CAD build for the part. Positions are in the model's coordinates, mm. Face numbers are marked on the shaded views. A direction names the side the tool comes from. Round coordinates to 2 decimals unless told otherwise and drop trailing zeros. Write each loop counter-clockwise with the first axis right and the second up, starting at its lowest first coordinate (ties: lowest second). Pieces come first, ordered by that corner, then holes. Notation, with made-up numbers: (17, -26) - (42, -26) arc R4 ccw to (42, -19) - close; hole circle Ø3 at (81, 47). An arc over 180 degrees is marked (long way). Answer in a Markdown table with one row per item.
```python
from build123d import *

# Parameters (mm, degrees)
F0_R     = 1.5875
F1_DEPTH = 38.1
F2_DEPTH = 40.64


with BuildPart() as f1:
    # F0 (on Front) → F1 (new body)
    with BuildSketch(Plane.XZ):
        with BuildLine():
            add(Edge.make_bspline(
                [(-2.039045, -1.229896), (-2.008193, -1.275858), (-1.977766, -1.322509), (-1.947774, -1.369864)],
                knots=[27.094619, 27.094619, 27.094619, 27.094619, 27.26278, 27.26278, 27.26278, 27.26278], degree=3))
            ThreePointArc((-2.039045, -1.229896), (-1.994638, -1.300681), (-1.947774, -1.369864))
        make_face()
        with BuildLine():
            add(Edge.make_bspline(
                [(2.019846, 1.26118), (2.011239, 1.274554), (2.002664, 1.287985), (1.994123, 1.301471)],
                knots=[27.195118, 27.195118, 27.195118, 27.195118, 27.242974, 27.242974, 27.242974, 27.242974], degree=3))
            ThreePointArc((1.994123, 1.301471), (1.133848, 2.093977), (0, 2.38125))
            ThreePointArc((0, 2.38125), (-2.073529, 1.170825), (-2.039045, -1.229896))
            add(Edge.make_bspline(
                [(-2.039045, -1.229896), (-2.008193, -1.275858), (-1.977766, -1.322509), (-1.947774, -1.369864)],
                knots=[27.094619, 27.094619, 27.094619, 27.094619, 27.26278, 27.26278, 27.26278, 27.26278], degree=3))
            ThreePointArc((-1.947774, -1.369864), (-1.133848, -2.093977), (-0.082606, -2.379817))
            ThreePointArc((-0.082606, -2.379817), (1.654335, -1.712755), (2.38125, 0))
            ThreePointArc((2.38125, 0), (2.289117, 0.65597), (2.019846, 1.26118))
        make_face()
        Circle(F0_R, mode=Mode.SUBTRACT)
    extrude(amount=F1_DEPTH)

    # F0 (on Front) → F2 (join)
    with BuildSketch(Plane.XZ):
        Circle(F0_R)
    extrude(amount=F2_DEPTH)


solid = f1.part
```
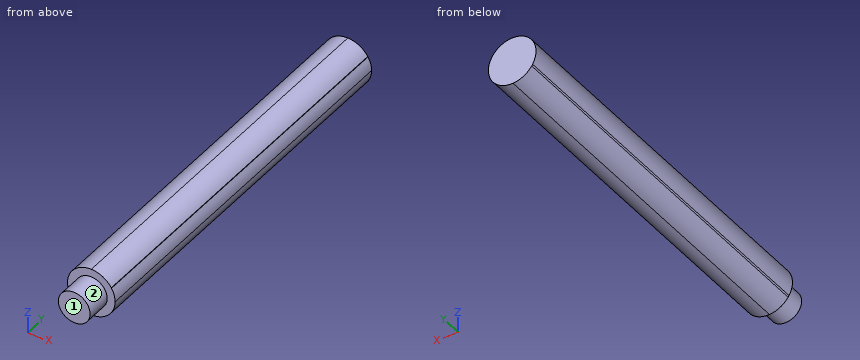
Q1. Flat gauge pin, fed straight in: pin 1 (1 mm diameter, centred on x = -1, y = -32, fed in from -Z). Where does the tip first touch, or does it go through?
Computed:
| item | result |
|---|---|
| pin 1 | stops at z = -2.33 |
Q2. Saw through at A-A on x = 1.2. List the corners of the cut face in (y, z).
Computed:
| item | result |
|---|---|
| outline | (-40.64, -1.04) - (-38.1, -1.04) - (-38.1, -2.06) - (0, -2.06) - (0, 2.06) - (-38.1, 2.06) - (-38.1, 1.04) - (-40.64, 1.04) - close |
Q3. Drill centre lines: line 1 (Y direction, x = 0.5, z = 1.65); line 2 (Z direction, x = -0.15, y = -25.5); line 3 (X direction, y = -19.5, z = -1.05). Where is each one in solid material? Low to high.
Computed:
| item | result |
|---|---|
| line 1 | y = -38.1 to 0 |
| line 2 | z = -2.38 to 2.38 |
| line 3 | x = -2.14 to 2.14 |
Q4. 3-axis set-ups, long thin cutter, end or side, ignore diameter. For the marked faces 1 and 2: which of +Z, -Z, +X, -X, +Y, -Y reach the whole face in a straight line?
Computed:
| item | result |
|---|---|
| face 1 | +Z, -Z, +X, -X, -Y |
| face 2 | -Y |
Q5. Saw through at C-C on z = -2. List the corners of the cut face in (x, y), then the cut area to 3 significant figures.
Computed:
| item | result |
|---|---|
| outline | (-1.29, -38.1) - (1.29, -38.1) - (1.29, 0) - (-1.29, 0) - close |
| area | 98.5 mm2 |
Q6. Saw through at B-B on z = 0.6. List the corners of the cut face in (x, y).
Computed:
| item | result |
|---|---|
| outline | (-2.3, -38.1) - (-1.47, -38.1) - (-1.47, -40.64) - (1.47, -40.64) - (1.47, -38.1) - (2.3, -38.1) - (2.3, 0) - (-2.3, 0) - close |
